For this review, use the dimensioned drawing (mm, ordinates from the lowest corner) and the shaded views. A direction names the side the tool comes from. Give positions to 0.01 mm unless a question says otherwise; leave off trailing zeros. Order: outer loops, then holes, each group sorted by start corner. A loop starts at its lowest first (then second) coordinate and runs counter-clockwise, first axis right, second up. Notation, with made-up numbers: M -26,8.5 L -20,8.5 A23 cw -20,40.5 Z; hole C -9.75,53 d7. An arc over 180 degrees is marked long. Answer as CSV lines item,"result". Start each with the question number.
1. Clearance check with flat-ended pins moving along their axes: P1, Ø3, axis at x = 3.5, z = 93, coming from the +Y side; P2, Ø1.5, axis at x = 2.5, y = 7, coming from the -Z side; P3, Ø1.8, axis at x = 2, y = 25, coming from the +Z side; P4, Ø2.5, axis at x = 3, z = 4.49, coming from the -Y side. State where each tip first meets the part, or that it passes through.
2. We need section C-C, the plane y = 6.5. Give the boundary of the cut face in (x, z), and give its area (3 significant figures).
3. For line 1 along Z through (x, y) = (3, 2.35); line 2 along Z through (x, y) = (3, 0.85); line 3 along Z through (x, y) = (3.45, 8), list the stretches that pass through material, from the lowest coordinate up.
4. We need section A-A, the plane z = 93.5. Give the boundary of the cut face in (x, y).
5. Machinability: for the marked faces 4, 5 and 6, which of the approach directions +Z, -Z, +X, -X, +Y, -Y give a long, thin tool a straight path to every point of the face, cutting with its end or side? Answer none if there is none.
6. We need section B-B, the plane y = 16.5. Give the boundary of the cut face in (x, z).
7. We need section D-D, the plane z = 80. Give the boundary of the cut face in (x, y).
8. Mouldability with a two-part tool opening along Z and no side actions: class the marked faces 1, 2 and 3 as pulls with the +Z half, pulls with the -Z half, needs draft (parallel to the pull), parting line crosses it, or undercut.
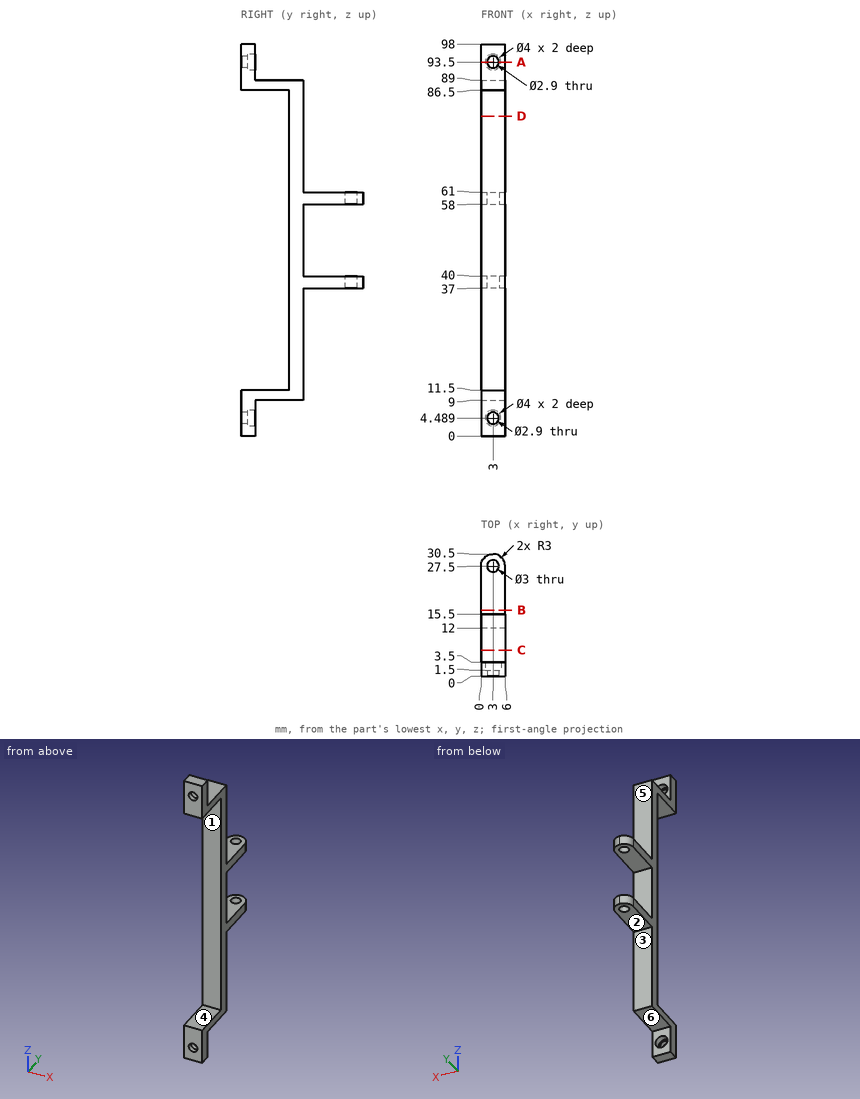
Result set:
1,P1,"y = 3.5"
1,P2,"z = 9"
1,P3,"z = 61"
1,P4,"through"
2,outline,"M 0,9 L 6,9 L 6,11.5 L 0,11.5 Z; M 0,86.5 L 6,86.5 L 6,89 L 0,89 Z"
2,area,"30.0 mm2"
3,line 1,"0 to 2.49, 6.49 to 11.5, 86.5 to 91.5, 95.5 to 98"
3,line 2,"0 to 3.04, 5.94 to 11.5, 86.5 to 92.05, 94.95 to 98"
3,line 3,"9 to 11.5, 86.5 to 89"
4,outline,"M 0,0 L 1.55,0 L 1.55,1.5 L 1,1.5 L 1,3.5 L 0,3.5 Z; M 4.45,0 L 6,0 L 6,3.5 L 5,3.5 L 5,1.5 L 4.45,1.5 Z"
5,face 4,"+X, -X, -Y"
5,face 5,"+Z, +X, -X, +Y"
5,face 6,"-Z, +X, -X, +Y"
6,outline,"M 0,37 L 6,37 L 6,40 L 0,40 Z; M 0,58 L 6,58 L 6,61 L 0,61 Z"
7,outline,"M 0,12 L 6,12 L 6,15.5 L 0,15.5 Z"
8,face 1,"undercut"
8,face 2,"pulls with the -Z half"
8,face 3,"needs draft"
